```python
from build123d import *

# Parameters (mm, degrees)
IZIM1_R                     = 1.25
Y_KSEKLIK_EKSTR_ZYON1_DEPTH = 50
IZIM2_R                     = 1.25
IZIM2_R_2                   = 0.75
KES_EKSTR_ZYON1_DEPTH       = 45
IZIM3_R                     = 1.75
Y_KSEKLIK_EKSTR_ZYON2_DEPTH = 3
IZIM4_R                     = 0.75
KES_EKSTR_ZYON2_DEPTH       = 4.5


with BuildPart() as part:
    # Çizim1 → Yükseklik-Ekstrüzyon1 (new body)
    with BuildSketch(Plane.XY):
        Circle(IZIM1_R)
    extrude(amount=Y_KSEKLIK_EKSTR_ZYON1_DEPTH)

    # Çizim2 → Kes-Ekstrüzyon1 (cut)
    with BuildSketch(Plane.XY.offset(50)):
        Circle(IZIM2_R)
        Circle(IZIM2_R_2, mode=Mode.SUBTRACT)
    extrude(amount=-KES_EKSTR_ZYON1_DEPTH, mode=Mode.SUBTRACT)

    # Çizim3 → Yükseklik-Ekstrüzyon2 (add)
    with BuildSketch(Plane.XY.offset(50)):
        Circle(IZIM3_R)
    extrude(amount=Y_KSEKLIK_EKSTR_ZYON2_DEPTH)

    # Çizim4 → Kes-Ekstrüzyon2 (cut, through all)
    with BuildSketch(Plane(origin=(1.75, 0, 0), x_dir=(0, 0, -1), z_dir=(1, 0, 0))):
        with Locations((-51.5, 0)):
            Circle(IZIM4_R)
    extrude(amount=-KES_EKSTR_ZYON2_DEPTH, mode=Mode.SUBTRACT)


solid = part.part
```
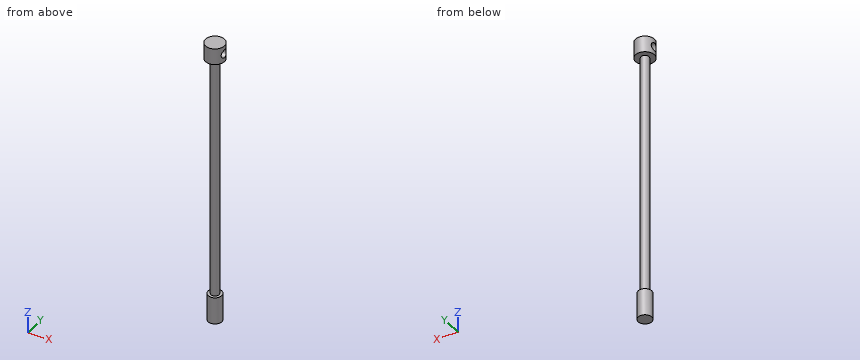
Geometry check sheet. Reference: the model listing, model coordinates, mm. Coordinates: 2 decimals unless noted, no trailing zeros. Order: outer loops, then holes, each group sorted by start corner. A loop starts at its lowest first (then second) coordinate and runs counter-clockwise, first axis right, second up. Notation, with made-up numbers: (57, -26) - (106, -26) arc R21 ccw to (106, 9) - close; hole circle Ø4 at (73.25, 7). An arc over 180 degrees is marked (long way). Answer as a JSON object with one key per item and string values. Group by question number.
Item 1: Sectioned sample at A-A, the plane x = 0. Record the cut outline in (y, z).
Item 2: Sectioned sample at B-B, the plane y = 0. Record the cut outline in (x, z).
Item 3: Depth check by flat-ended pin: pin 1 Ø1.5 at (y, z) = (-1, 13) entering from -X. Enter the tip coordinate at first touch or a pass-through.
Item 4: Sectioned sample at D-D, the plane z = 11.5. Record the cut outline in (x, y).
Item 5: Sectioned sample at C-C, the plane z = 51.5. Record the cut outline in (x, y), and give its area (3 significant figures).
Item 6: Scan lines: probe 1 along Z at (x, y) = (0.2, 0); probe 2 along Z at (x, y) = (-0.95, 0.25); probe 3 along Z at (x, y) = (-0.45, -1). Record each from-to range of solid material in increasing order.
Resolved:
{
 "1": {"outline": "(-1.75, 50) - (-0.75, 50) - (-0.75, 5) - (-1.25, 5) - (-1.25, 0) - (1.25, 0) - (1.25, 5) - (0.75, 5) - (0.75, 50) - (1.75, 50) - (1.75, 53) - (-1.75, 53) - close; hole circle Ø1.5 at (0, 51.5)"},
 "2": {"outline": "(-1.75, 50) - (-0.75, 50) - (-0.75, 5) - (-1.25, 5) - (-1.25, 0) - (1.25, 0) - (1.25, 5) - (0.75, 5) - (0.75, 50) - (1.75, 50) - (1.75, 50.75) - (-1.75, 50.75) - close; (-1.75, 52.25) - (1.75, 52.25) - (1.75, 53) - (-1.75, 53) - close"},
 "3": {"pin 1": "x = -0.71"},
 "4": {"outline": "circle Ø1.5 at (0, 0)"},
 "5": {"outline": "(-1.58, -0.75) arc R1.75 ccw to (1.58, -0.75) - close; (-1.58, 0.75) - (1.58, 0.75) arc R1.75 ccw to start", "area": "4.54 mm^2"},
 "6": {"probe 1": "0 to 50.75, 52.25 to 53", "probe 2": "0 to 5, 50 to 50.79, 52.21 to 53", "probe 3": "0 to 5, 50 to 53"}
}
